Read the model definition and answer for the solid it produces. Units are mm, in the model's axes. A direction names the side the tool comes from. Coordinates: 2 decimals unless noted, no trailing zeros. Write each loop counter-clockwise with the first axis right and the second up, starting at its lowest first coordinate (ties: lowest second). Pieces come first, ordered by that corner, then holes. Notation, with made-up numbers: (-9.75, -6) -> (2.25, -6) arc R8 ccw to (2.25, 3) -> close; hole circle Ø6 at (37, -18). An arc over 180 degrees is marked (long way). Write item = value, one per line. Start each with the question number.
1) Section A-A (z = 1.65) is taken. Count the separate pieces of the cut face and the enclosed holes in it, plus the area to 3 significant figures.
2) For a pull along X with two mould halves and no side action, classify faces 3 (the face through (73.986, 5.703, 1.541)), 4 (the face through (61.24, 34.58, 1.54)), 5 (the face through (26, 88, 2)) as released by +X, released by -X, zero draft, split by the parting line, or undercut.
3) Section B-B (x = 72) is taken. Determine the outline of the cut face in (y, z) (3 decimals).
4) Section D-D (y = 27.5) is taken. Determine the outline of the cut face in (x, z) (3 decimals), plus the area to 3 significant figures.
5) Find the intervals of material crossed by line 1 along Y through (x, z) = (29.5, 2); line 2 along Y through (x, z) = (10, 1.4); line 3 along X through (y, z) = (40, 0.3), in increasing order. Write a range as from..to.
6) Section C-C (y = 73) is taken. Determine the outline of the cut face in (x, z) (3 decimals).
7) A tool of negligible diameter and unlimited length cuts with its end or side. For faces 1 (the face through (5.561, 73, 2)), 2 (the face through (70.019, 77.475, 1.541)), from which of +Z, -Z, +X, -X, +Y, -Y can it reach the whole face along a straight path? Write none if from no direction.
8) Flat-ended cylindrical pins translate along their axes: pin 1 Ø3 at (x, y) = (10, 53) entering from -Z; pin 2 Ø1 at (y, z) = (75, 1.5) entering from +X; pin 3 Ø0.9 at (x, z) = (3.5, 1.5) entering from -Y. Find the tip coordinate at first contact, or state that the pin passes through.
from build123d import *

# Parameters (mm, degrees)
MODEL_R             = 2.6
MODEL_R_2           = 12
MODEL_R_3           = 1.6
MODEL_R_4           = 3.675
MODEL_W             = 3.760660172
MODEL_H             = 11
BOSS_EXTRUDE1_DEPTH = 3.125


with BuildPart() as part:
    # Model → Boss-Extrude1 (new body)
    with BuildSketch(Plane.XY):
        with BuildLine():
            Line((80, 20), (80, 53))
            ThreePointArc((80, 53), (69.748737342, 77.748737342), (45, 88))
            Line((45, 88), (7, 88))
            ThreePointArc((7, 88), (2.050252532, 85.949747468), (0, 81))
            Line((0, 81), (0, 20))
            ThreePointArc((0, 20), (5.857864376, 5.857864376), (20, 0))
            Line((20, 0), (60, 0))
            ThreePointArc((60, 0), (74.142135624, 5.857864376), (80, 20))
        make_face()
        with Locations((10, 73)):
            Circle(MODEL_R, mode=Mode.SUBTRACT)
        with Locations((45, 20.5)):
            Circle(MODEL_R_2, mode=Mode.SUBTRACT)
        with Locations((18, 39)):
            Circle(MODEL_R, mode=Mode.SUBTRACT)
        with Locations((60.5, 36)):
            Circle(MODEL_R_3, mode=Mode.SUBTRACT)
        with Locations((29.5, 5)):
            Circle(MODEL_R_3, mode=Mode.SUBTRACT)
        with Locations((45, 79)):
            Circle(MODEL_R_4, mode=Mode.SUBTRACT)
        with Locations((10, 53)):
            Circle(MODEL_R, mode=Mode.SUBTRACT)
        with Locations((29.5, 36)):
            Circle(MODEL_R_3, mode=Mode.SUBTRACT)
        with Locations((60.5, 5)):
            Circle(MODEL_R_3, mode=Mode.SUBTRACT)
        with Locations((72, 39)):
            Circle(MODEL_R, mode=Mode.SUBTRACT)
        with Locations((3.680330086, 73)):
            Rectangle(MODEL_W, MODEL_H, mode=Mode.SUBTRACT)
    extrude(amount=BOSS_EXTRUDE1_DEPTH)


solid = part.part
Answer key:
q1.separate_pieces = 1
q1.enclosed_holes = 11
q1.area = 5,940 mm^2
q2.face_3 = released by +X
q2.face_4 = undercut
q2.face_5 = zero draft
q3.outline = (4, 0) -> (36.4, 0) -> (36.4, 3.125) -> (4, 3.125) -> close; (41.6, 0) -> (75.271, 0) -> (75.271, 3.125) -> (41.6, 3.125) -> close
q4.outline = (0, 0) -> (35.253, 0) -> (35.253, 3.125) -> (0, 3.125) -> close; (54.747, 0) -> (80, 0) -> (80, 3.125) -> (54.747, 3.125) -> close
q4.area = 189 mm^2
q5.line_1 = 0..3.4, 6.6..34.4, 37.6..88
q5.line_2 = 2.68..50.4, 55.6..70.4, 75.6..88
q5.line_3 = 0..15.6, 20.4..69.6, 74.4..80
q6.outline = (0, 0) -> (1.8, 0) -> (1.8, 3.125) -> (0, 3.125) -> close; (5.561, 0) -> (7.4, 0) -> (7.4, 3.125) -> (5.561, 3.125) -> close; (12.6, 0) -> (73.723, 0) -> (73.723, 3.125) -> (12.6, 3.125) -> close
q7.face_1 = +Z, -Z
q7.face_2 = +Z, -Z, +X, +Y
q8.pin_1 = through
q8.pin_2 = 72.62
q8.pin_3 = 8.07
